For this review, take the finished solid that the model builds, in its own axes (mm). A direction names the side the tool comes from. Give positions to 0.01 mm unless a question says otherwise; leave off trailing zeros. Loops run counter-clockwise (first coordinate to the right, second up) from the corner with the lowest first, then second, coordinate; pieces in that order, holes last. Notation, with made-up numbers: (11, 14) -> (33, 14) arc R20 cw to (33, 23) -> close; hole circle Ø8 at (16, -27). An arc over 180 degrees is marked (long way). One line per question, with ' | ' between items. Start each with the question number.
(1) Tool access review of faces 4 (the flat face through (-1, 2197, -1)), 5 (the flat face through (-1, 2200, -1)): name each direction out of +Z, -Z, +X, -X, +Y, -Y from which nothing blocks a thin tool from reaching the whole face with its end or side.
(2) Consider section A-A (x = 0). Write out the cut boundary in (y, z), and give its area (3 significant figures).
(3) Wall thickness on probe 1 along Y at (x, z) = (-14.5, 37.5); probe 2 along X at (y, z) = (1741, -36): over which ranges is each line inside the solid? List them lowest first.
(4) Consider section D-D (y = 1031.5). Write out the cut boundary in (x, z).
(5) Draft analysis for pull direction Z (two halves, no side actions). For faces 1 (the flat face through (-50, 1085, 1)), 2 (the flat face through (-1, 1085, 50)), 3 (the flat face through (-47, 1085, 1)), state which applies: +Z half, -Z half, draft (parallel to the pull), parting line (faces both ways), or undercut.
(6) Consider section B-B (y = 1896.5). Write out the cut boundary in (x, z), and give its area (3 significant figures).
(7) Consider section C-C (z = -17.5). Write out the cut boundary in (x, y), and give its area (3 significant figures).
from build123d import *

# Parameters (mm, degrees)
SKETCH1_W           = 100
SKETCH1_H           = 100
BOSS_EXTRUDE1_DEPTH = 2200
SHELL1_T            = 3
CUT_EXTRUDE2_DEPTH  = 10


with BuildPart() as part:
    # Sketch1 → Boss-Extrude1 (new body)
    with BuildSketch(Plane(origin=(0, 0, 0), x_dir=(1, 0, 0), z_dir=(0, 1, 0))):
        Rectangle(SKETCH1_W, SKETCH1_H)
    extrude(amount=BOSS_EXTRUDE1_DEPTH)

    # Shell1 (no face opened: a closed hollow body)
    add(offset(amount=-SHELL1_T, mode=Mode.PRIVATE), mode=Mode.SUBTRACT)

    # Sketch3 → Cut-Extrude2 (cut)
    with BuildSketch(Plane(origin=(0, 0, -50), x_dir=(-1, 0, 0), z_dir=(0, 0, -1))):
        with BuildLine():
            Line((-25, 350), (-25, 1850))
            ThreePointArc((-25, 1850), (0, 1875), (25, 1850))
            Line((25, 1850), (25, 350))
            ThreePointArc((25, 350), (0, 325), (-25, 350))
        make_face()
    extrude(amount=-CUT_EXTRUDE2_DEPTH, mode=Mode.SUBTRACT)


solid = part.part
A:
1) face 4: none | face 5: +Z, -Z, +X, -X, +Y
2) outline: (0, -50) -> (325, -50) -> (325, -47) -> (3, -47) -> (3, 47) -> (2197, 47) -> (2197, -47) -> (1875, -47) -> (1875, -50) -> (2200, -50) -> (2200, 50) -> (0, 50) -> close | area: 9,110 mm^2
3) probe 1: y = 0 to 3, 2197 to 2200 | probe 2: x = -50 to -47, 47 to 50
4) outline: (-50, -50) -> (-25, -50) -> (-25, -47) -> (-47, -47) -> (-47, 47) -> (47, 47) -> (47, -47) -> (25, -47) -> (25, -50) -> (50, -50) -> (50, 50) -> (-50, 50) -> close
5) face 1: draft | face 2: +Z half | face 3: undercut
6) outline: (-50, -50) -> (50, -50) -> (50, 50) -> (-50, 50) -> close; hole (-47, -47) -> (47, -47) -> (47, 47) -> (-47, 47) -> close | area: 1,160 mm^2
7) outline: (-50, 0) -> (50, 0) -> (50, 2200) -> (-50, 2200) -> close; hole (-47, 3) -> (47, 3) -> (47, 2197) -> (-47, 2197) -> close | area: 13,800 mm^2
